For this review, take the finished solid that the model builds, in its own axes (mm). A direction names the side the tool comes from. Give positions to 0.01 mm unless a question says otherwise; leave off trailing zeros. Loops run counter-clockwise (first coordinate to the right, second up) from the corner with the lowest first, then second, coordinate; pieces in that order, holes last.
```python
from build123d import *

# Parameters (mm, degrees)
F0_W      = 38.1
F0_H      = 38.1
F1_DEPTH  = 38.1
F6_DEPTH  = 76.2
F8_DEPTH  = 76.2
F9_W      = 25.4
F9_H      = 7.62
F10_DEPTH = 76.2


with BuildPart() as f1:
    # F0 (on Front) → F1 (new body)
    with BuildSketch(Plane.XZ):
        with Locations((-19.05, 19.05)):
            Rectangle(F0_W, F0_H)
    extrude(amount=F1_DEPTH)

    # F5 (on offset) → F6 (cut)
    with BuildSketch(Plane.YZ.offset(38.1)):
        Polygon((-11.43, 15.2127137408), (-6.35, 38.1), (-31.75, 38.1), (-26.67, 15.3867928311), (-21.59, 28.0867928311), (-16.51, 28.0867928311), align=None)
        Polygon((-31.75, 0), (-38.1, 38.1), (-38.1, 0), align=None)
        Polygon((-25.4, 0), (-12.7, 0), (-19.05, 15.875), align=None)
        Polygon((-6.35, 0), (0, 0), (0, 38.1), align=None)
    extrude(amount=-F6_DEPTH, mode=Mode.SUBTRACT)

    # F7 (on offset) → F8 (cut)
    with BuildSketch(Plane.XZ.offset(38.1)):
        Polygon((-19.05, 22.225), (-12.7, 38.1), (-25.4, 38.1), align=None)
        Polygon((-38.1, 38.1), (-38.1, 0), (-31.75, 38.1), align=None)
        Polygon((-31.75, 0), (-6.35, 0), (-11.43, 22.225), (-16.51, 9.525), (-21.59, 9.525), (-26.67, 22.225), align=None)
        Polygon((-6.35, 38.1), (0, 0), (0, 38.1), align=None)
    extrude(amount=-F8_DEPTH, mode=Mode.SUBTRACT)

    # F9 (on offset) → F10 (cut)
    with BuildSketch(Plane.XY.offset(38.1)):
        with Locations((-25.4, -26.67)):
            Rectangle(F9_W, F9_H)
        with Locations((-12.7, -11.43)):
            Rectangle(F9_W, F9_H)
    extrude(amount=-F10_DEPTH, mode=Mode.SUBTRACT)


solid = f1.part
```
Item 1: Take a section at B-B on x = -12. Give the boundary of the cut face in (y, z), and give its area (3 significant figures).
Answer:
outline: (-38.1, 38.1) - (-35.22, 20.8) - (-27.88, 20.8) - (-31.75, 38.1) - close; (-24.5, 20.8) - (-15.24, 20.8) - (-15.24, 24.87) - (-16.51, 28.09) - (-21.59, 28.09) - close; (-7.62, 20.8) - (-2.88, 20.8) - (0, 38.1) - (-6.35, 38.1) - (-7.62, 32.38) - close
area: 276 mm2
Item 2: Take a section at A-A on z = 27. Give the boundary of the cut face in (x, y).
Answer:
outline: (-33.6, -36.25) - (-20.96, -36.25) - (-20.96, -30.48) - (-33.6, -30.48) - close; (-33.6, -22.02) - (-20.96, -22.02) - (-20.96, -16.08) - (-33.6, -16.08) - close; (-33.6, -8.81) - (-25.4, -8.81) - (-25.4, -7.62) - (-20.96, -7.62) - (-20.96, -1.85) - (-33.6, -1.85) - close; (-17.14, -36.25) - (-4.5, -36.25) - (-4.5, -29.27) - (-12.7, -29.27) - (-12.7, -30.48) - (-17.14, -30.48) - close; (-17.14, -22.02) - (-4.5, -22.02) - (-4.5, -16.08) - (-17.14, -16.08) - close; (-17.14, -7.62) - (-4.5, -7.62) - (-4.5, -1.85) - (-17.14, -1.85) - close
Item 3: Clearance check with flat-ended pins moving along their axes: pin 1 Ø12.5 at (x, z) = (-23, 9.5) entering from +Y (3 decimals); pin 2 Ø10 at (x, y) = (-10.5, -30.5) entering from +Z; pin 3 Ø0.9 at (y, z) = (-28.5, 24.5) entering from -X; pin 4 Ø8 at (x, y) = (-15.5, -29.5) entering from -Z (3 decimals). State where each tip first meets the part, or that it passes through.
Answer:
pin 1: stops at y = -3.725
pin 2: stops at z = 38.1
pin 3: stops at x = -12.7
pin 4: stops at z = 9.525
Item 4: The part is to be moulded in two halves that separate along Y. For faces 5 (the flat face through (-19, -20, 13.5)), 6 (the flat face through (-29, -3, 38.1)), say which applies: released by +Y, released by -Y, zero draft, split by the parting line, or undercut.
Answer:
face 5: undercut
face 6: zero draft
Item 5: For L1, parallel to X at y = -17, z = 15; L2, parallel to Y at x = -14, z = 25.5; L3, parallel to X at y = -16.5, z = 10, list the stretches that pass through material, from the lowest coordinate up.
Answer:
L1: x = -35.6 to -28.32, -23.78 to -14.32, -9.78 to -2.5
L2: y = -36 to -30.48, -22.62 to -15.49, -7.62 to -2.1
L3: x = -36.43 to -29.46, -21.78 to -16.32, -8.64 to -1.67
Item 6: Tool access review of faces 1 (the flat face through (-5.5, -17.1, 11)), 2 (the flat face through (-10.972, -15.884, 26.5)), 3 (the flat face through (-22.27, -33.5, 30.27)), 4 (the flat face through (-19, -22, 9.525)): name each direction out of +Z, -Z, +X, -X, +Y, -Y from which nothing blocks a thin tool from reaching the whole face with its end or side.
Answer:
face 1: -Z, +X, -X
face 2: +Z, +X, -X
face 3: +Z, +Y, -Y
face 4: -Z, +Y, -Y
Item 7: Take a section at D-D on z = 35.5. Give the boundary of the cut face in (x, y).
Answer:
outline: (-32.18, -37.67) - (-24.36, -37.67) - (-24.36, -31.17) - (-32.18, -31.17) - close; (-32.18, -6.93) - (-24.36, -6.93) - (-24.36, -0.43) - (-32.18, -0.43) - close; (-13.74, -37.67) - (-5.92, -37.67) - (-5.92, -31.17) - (-13.74, -31.17) - close; (-13.74, -6.93) - (-5.92, -6.93) - (-5.92, -0.43) - (-13.74, -0.43) - close
Item 8: Take a section at C-C on y = -3.5. Give the boundary of the cut face in (x, z) (3 decimals).
Answer:
outline: (-35.25, 17.1) - (-27.841, 17.1) - (-26.67, 22.225) - (-24.62, 17.1) - (-13.48, 17.1) - (-11.43, 22.225) - (-10.259, 17.1) - (-2.85, 17.1) - (-6.35, 38.1) - (-12.7, 38.1) - (-19.05, 22.225) - (-25.4, 38.1) - (-31.75, 38.1) - close
